Design review of the part built by this model. Coordinates are the model's own, in mm. A direction names the side the tool comes from. Round coordinates to 2 decimals unless told otherwise and drop trailing zeros. Write each loop counter-clockwise with the first axis right and the second up, starting at its lowest first coordinate (ties: lowest second). Pieces come first, ordered by that corner, then holes. Notation, with made-up numbers: M 47,76.25 L 104,76.25 A17 cw 104,107.25 Z; hole C 51,65 d10. An arc over 180 degrees is marked long. One line per question, with ' | ' between items. Start each with the question number.
Item 1: Add section A-A, the plane y = 58. State the section outline as (x, z) points, and give its area (3 significant figures).
Item 2: Add section C-C, the plane x = -69. State the section outline as (y, z) points.
Item 3: For L1, parallel to X at y = 34, z = -3.75; L2, parallel to Y at x = -94, z = -2.25; L3, parallel to Y at x = -14, z = 4.75, list the stretches that pass through material, from the lowest coordinate up.
Item 4: Machinability: for faces 5 (the face through (-12, 46, 1)), 6 (the face through (-14.792, 23, -1)), 7 (the face through (-107, 43, -2.492)), which of the approach directions +Z, -Z, +X, -X, +Y, -Y give a long, thin tool a straight path to every point of the face, cutting with its end or side? Answer none if there is none.
Item 5: Draft analysis for pull direction X (two halves, no side actions). For faces 1 (the face through (-92.292, 43, 0)), 2 (the face through (-9, 23, -0.042)), 3 (the face through (-72.292, 45, -4)), 4 (the face through (-20.292, 41, -1)), state which applies: released by +X, released by -X, zero draft, split by the parting line, or undercut.
Item 6: Add section B-B, the plane y = 37. State the section outline as (x, z) points.
Item 7: Insertion check: pin 1 Ø1.7 at (y, z) = (37, -8.5) entering from -X; pin 2 Ø8 at (y, z) = (56.5, -7) entering from +X; pin 3 Ø5 at (x, z) = (-98.5, 4.5) entering from +Y. Each pin has a flat end and moves straight along its axis. Give the tip position at first contact, or say it passes through.
```python
from build123d import *

# Parameters (mm, degrees)
BOSS_EXTRUDE1_DEPTH = 20
FILLET1_R           = 1
SKETCH2_R           = 9
CUT_EXTRUDE1_DEPTH  = 20
BOSS_EXTRUDE2_START = 2
BOSS_EXTRUDE2_DEPTH = 2
SKETCH4_W           = 20
SKETCH4_H           = 20
BOSS_EXTRUDE3_DEPTH = 2
FILLET2_R           = 1
SKETCH5_W           = 12.5
SKETCH5_H           = 2
CUT_EXTRUDE2_DEPTH  = 24
BOSS_EXTRUDE4_DEPTH = 80
FILLET3_R           = 1
SKETCH8_R           = 7.11392485
SKETCH8_W           = 20
SKETCH8_H           = 40
CUT_EXTRUDE3_DEPTH  = 2
SKETCH9_W           = 20
SKETCH9_H           = 2
BOSS_EXTRUDE5_DEPTH = 16
FILLET4_R           = 1
SKETCH10_R          = 2.5
CUT_EXTRUDE4_DEPTH  = 20
CUT_EXTRUDE5_DEPTH  = 1000
SKETCH16_W          = 44.924413541
SKETCH16_H          = 28.761805837
CUT_EXTRUDE6_DEPTH  = 200


with BuildPart() as part:
    # Sketch1 → Boss-Extrude1 (new body)
    with BuildSketch(Plane(origin=(0, 0, 0), x_dir=(1, 0, 0), z_dir=(0, 1, 0))):
        Polygon((-2.291666667, 11.041666667), (-22.291666667, 11.041666667), (-22.291666667, -8.958333333), (-2.291666667, -8.958333333), (-2.291666667, -6.958333333), (-20.291666667, -6.958333333), (-20.291666667, 9.041666667), (-2.291666667, 9.041666667), align=None)
    extrude(amount=BOSS_EXTRUDE1_DEPTH)

    # Fillet1
    fillet1_edges = [part.edges().sort_by_distance(p)[0] for p in [
        (-22.291666667, 10, 8.958333333),
        (-22.291666667, 10, -11.041666667),
    ]]
    fillet(fillet1_edges, radius=FILLET1_R)

    # Sketch2 → Cut-Extrude1 (cut)
    with BuildSketch(Plane.XY.offset(8.958333333)):
        with Locations(Location((-12.291666667, 10, 0), (0, 0, 180))):
            Circle(SKETCH2_R)
    extrude(amount=-CUT_EXTRUDE1_DEPTH, mode=Mode.SUBTRACT)

    # Sketch3 → Boss-Extrude2 (add)
    with BuildSketch(Plane(origin=(0, 20, 0), x_dir=(1, 0, 0), z_dir=(0, 1, 0)).offset(BOSS_EXTRUDE2_START)):
        Polygon((-2.291666667, 2.377848536), (-2.291666667, 9.041666667), (-20.291666667, 9.041666667), (-20.291666667, -6.958333333), (-2.291666667, -6.958333333), (-2.291666667, 0.377848536), align=None)
        with BuildLine():
            Line((-2.291666667, 9.041666667), (-2.291666667, 11.041666667))
            Line((-2.291666667, 11.041666667), (-21.291666667, 11.041666667))
            ThreePointArc((-21.291666667, 11.041666667), (-21.998773448, 10.748773448), (-22.291666667, 10.041666667))
            Line((-22.291666667, 10.041666667), (-22.291666667, -7.958333333))
            ThreePointArc((-22.291666667, -7.958333333), (-21.998773448, -8.665440115), (-21.291666667, -8.958333333))
            Line((-21.291666667, -8.958333333), (-2.291666667, -8.958333333))
            Line((-2.291666667, -8.958333333), (-2.291666667, -6.958333333))
            Line((-2.291666667, -6.958333333), (-20.291666667, -6.958333333))
            Line((-20.291666667, -6.958333333), (-20.291666667, 9.041666667))
            Line((-20.291666667, 9.041666667), (-2.291666667, 9.041666667))
        make_face()
    extrude(amount=-BOSS_EXTRUDE2_DEPTH)

    # Sketch4 → Boss-Extrude3 (add)
    with BuildSketch(Plane.XZ):
        with Locations((-12.291666667, -1.041666667)):
            Rectangle(SKETCH4_W, SKETCH4_H)
    extrude(amount=BOSS_EXTRUDE3_DEPTH)

    # Fillet2
    fillet2_edges = [part.edges().sort_by_distance(p)[0] for p in [
        (-22.291666667, -1, -11.041666667),
        (-22.291666667, -1, 8.958333333),
    ]]
    fillet(fillet2_edges, radius=FILLET2_R - 0.0001)  # a hair under: the kernel refuses the full size

    # Sketch5 → Cut-Extrude2 (cut)
    with BuildSketch(Plane(origin=(0, 22, 0), x_dir=(1, 0, 0), z_dir=(0, 1, 0))):
        with Locations((-8.541666667, 1.041666667)):
            Rectangle(SKETCH5_W, SKETCH5_H)
    extrude(amount=-CUT_EXTRUDE2_DEPTH, mode=Mode.SUBTRACT)

    # Sketch6 → Boss-Extrude4 (add)
    with BuildSketch(Plane.ZY.offset(22.291666667)):
        Polygon((-2.491666667, -37), (-4.491666667, -37), (-4.491666667, -2), (-4.491666667, 22), (-2.491666667, 22), (-2.491666667, -2), align=None)
    extrude(amount=BOSS_EXTRUDE4_DEPTH)

    # Fillet3
    fillet3_edges = [part.edges().sort_by_distance(p)[0] for p in [
        (-22.291666667, -37, -3.491666667),
        (-102.291666667, 22, -3.491666667),
        (-102.291666667, -37, -3.491666667),
    ]]
    fillet(fillet3_edges, radius=FILLET3_R)

    # Sketch8 → Cut-Extrude3 (cut)
    with BuildSketch(Plane(origin=(0, 0, -4.491666667), x_dir=(-1, 0, 0), z_dir=(0, 0, -1))):
        with Locations((12.291666667, 10)):
            Circle(SKETCH8_R)
        with Locations((82.291666667, -1)):
            Rectangle(SKETCH8_W, SKETCH8_H)
    extrude(amount=-CUT_EXTRUDE3_DEPTH, mode=Mode.SUBTRACT)

    # Sketch9 → Boss-Extrude5 (add)
    with BuildSketch(Plane.XY.offset(-2.491666667)):
        Polygon((-92.823958121, 20), (-112.291666667, 20), (-112.291666667, 18), (-92.291666667, 18), (-92.291666667, 20), align=None)
        with Locations((-102.291666667, 1)):
            Rectangle(SKETCH9_W, SKETCH9_H)
    extrude(amount=BOSS_EXTRUDE5_DEPTH)

    # Fillet4
    fillet4_edges = [part.edges().sort_by_distance(p)[0] for p in [
        (-112.291666667, 19, -2.491666667),
        (-112.291666667, 19, 13.508333333),
        (-92.291666667, 19, 13.508333333),
        (-112.291666667, 1, -2.491666667),
        (-92.291666667, 1, 13.508333333),
        (-112.291666667, 1, 13.508333333),
    ]]
    fillet(fillet4_edges, radius=FILLET4_R)

    # Sketch10 → Cut-Extrude4 (cut)
    with BuildSketch(Plane(origin=(0, 20, 0), x_dir=(1, 0, 0), z_dir=(0, 1, 0))):
        with Locations(Location((-97.291666667, -5.508333333, 0), (0, 0, 180))):
            Circle(SKETCH10_R)
        with Locations(Location((-107.291666667, -5.508333333, 0), (0, 0, 180))):
            Circle(SKETCH10_R)
    extrude(amount=-CUT_EXTRUDE4_DEPTH, mode=Mode.SUBTRACT)

    # Mirror18: part across plane


with BuildPart() as part_1:
    add(part.part)
    add(part.part.mirror(Plane.ZX.offset(22)))

    # Sketch15 → Cut-Extrude5 (cut)
    with BuildSketch(Plane.ZY.offset(102.291666667)):
        Polygon((-4.491666667, 22), (26.371176894, 22), (26.371176894, -60.225143759), (-46.701352218, -60.225143759), (-46.701352218, 21.5), align=None)
    extrude(amount=-CUT_EXTRUDE5_DEPTH, mode=Mode.SUBTRACT)


with BuildPart() as cut_extrude5_piece_1:
    # of the separate pieces the step leaves, piece 1, a body of its own (cut_extrude5_pieces)
    add(part_1.part.solids().sort_by_distance((-101.291666667, 22, -2.491666667))[0])


with BuildPart() as cut_extrude5_piece_2:
    # of the separate pieces the step leaves, piece 2, a body of its own (cut_extrude5_pieces)
    add(part_1.part.solids().sort_by_distance((-112.291666667, 20, -1.491666667))[0])


with BuildPart() as cut_extrude5_piece_3:
    # of the separate pieces the step leaves, piece 3, a body of its own (cut_extrude5_pieces)
    add(part_1.part.solids().sort_by_distance((-111.291666667, 2, -2.491666667))[0])


with BuildPart() as cut_extrude6_tool:
    # Sketch16 → Cut-Extrude6 (new body)
    with BuildSketch(Plane(origin=(-102.291666667, 0, 0), x_dir=(0, 0, -1), z_dir=(1, 0, 0))):
        with Locations((-5.305801417, 7.602093766)):
            Rectangle(SKETCH16_W, SKETCH16_H)
    extrude(amount=-CUT_EXTRUDE6_DEPTH)


with BuildPart() as cut_extrude5_piece_2_1:
    add(cut_extrude5_piece_2.part)

    # Cut-Extrude6: cut by cut_extrude6_tool
    add(cut_extrude6_tool.part, mode=Mode.SUBTRACT)


with BuildPart() as cut_extrude5_piece_3_1:
    add(cut_extrude5_piece_3.part)

    # Cut-Extrude6: cut by cut_extrude6_tool
    add(cut_extrude6_tool.part, mode=Mode.SUBTRACT)


solid = cut_extrude5_piece_1.part
```
Computed values:
1) outline: M -102.29,-4.49 L -92.29,-4.49 L -92.29,-2.49 L -102.29,-2.49 Z; M -72.29,-4.49 L -22.29,-4.49 L -22.29,-2.49 L -72.29,-2.49 Z | area: 120 mm^2
2) outline: M 22,-4.49 L 81,-4.49 L 81,-2.49 L 22,-2.49 Z
3) L1: x = -102.29 to -92.29, -72.29 to -21.29 | L2: y = 24 to 26, 42 to 44 | L3: y = 22 to 24, 44 to 46
4) face 5: +Z, -Z, +X, +Y | face 6: +X, +Y, -Y | face 7: -Z, -X, +Y, -Y
5) face 1: undercut | face 2: zero draft | face 3: undercut | face 4: released by +X
6) outline: M -102.29,-4.49 L -92.29,-4.49 L -92.29,-2.49 L -102.29,-2.49 Z; M -72.29,-4.49 L -22.29,-4.49 L -22.29,-10.04 A1 ccw -21.29,-11.04 L -20.78,-11.04 L -20.78,8.96 L -21.29,8.96 A1 ccw -22.29,7.96 L -22.29,-2.49 L -72.29,-2.49 Z; M -3.81,-11.04 L -2.29,-11.04 L -2.29,-9.04 L -3.81,-9.04 Z; M -3.81,6.96 L -2.29,6.96 L -2.29,8.96 L -3.81,8.96 Z
7) pin 1: stops at x = -22.29 | pin 2: stops at x = -22.29 | pin 3: stops at y = 44
